Job drawing, mm, ordinate dimensions from the low corner. One solid piece. Round coordinates to 2 decimals unless told otherwise and drop trailing zeros. Write each loop counter-clockwise with the first axis right and the second up, starting at its lowest first coordinate (ties: lowest second). Pieces come first, ordered by that corner, then holes.
1) Saw through at B-B (x = 50). Write the cut outline in (y, z), plus the area to 3 significant figures.
2) Saw through at C-C (y = 89). Write the cut outline in (x, z), plus the area to 3 significant figures.
3) Wall check: probe 1 along Z at (x, y) = (19, 71.5); probe 2 along Y at (x, z) = (61.5, 37); probe 3 along Y at (x, z) = (26, 64) (1 decimal). Give the ranges that are in metal, low to high.
4) Flat gauge pins, fed straight in: pin 1 (1.8 mm diameter, centred on x = 19, y = 136.5, fed in from +Z); pin 2 (3 mm diameter, centred on x = 52.5, z = 20, fed in from -Y); pin 3 (8 mm diameter, centred on x = 26, y = 30, fed in from +Z). Where does each tip first touch, or does it go through?
5) Saw through at A-A (z = 33). Write the cut outline in (x, y), plus the area to 3 significant figures.
6) Saw through at D-D (z = 21.5). Write the cut outline in (x, y).
7) Pull direction Y, two halves, no side cores. Call the marked faces 1, 2, 3 and 4: +Y half, -Y half, draft (parallel to the pull), parting line (faces both ways), or undercut.
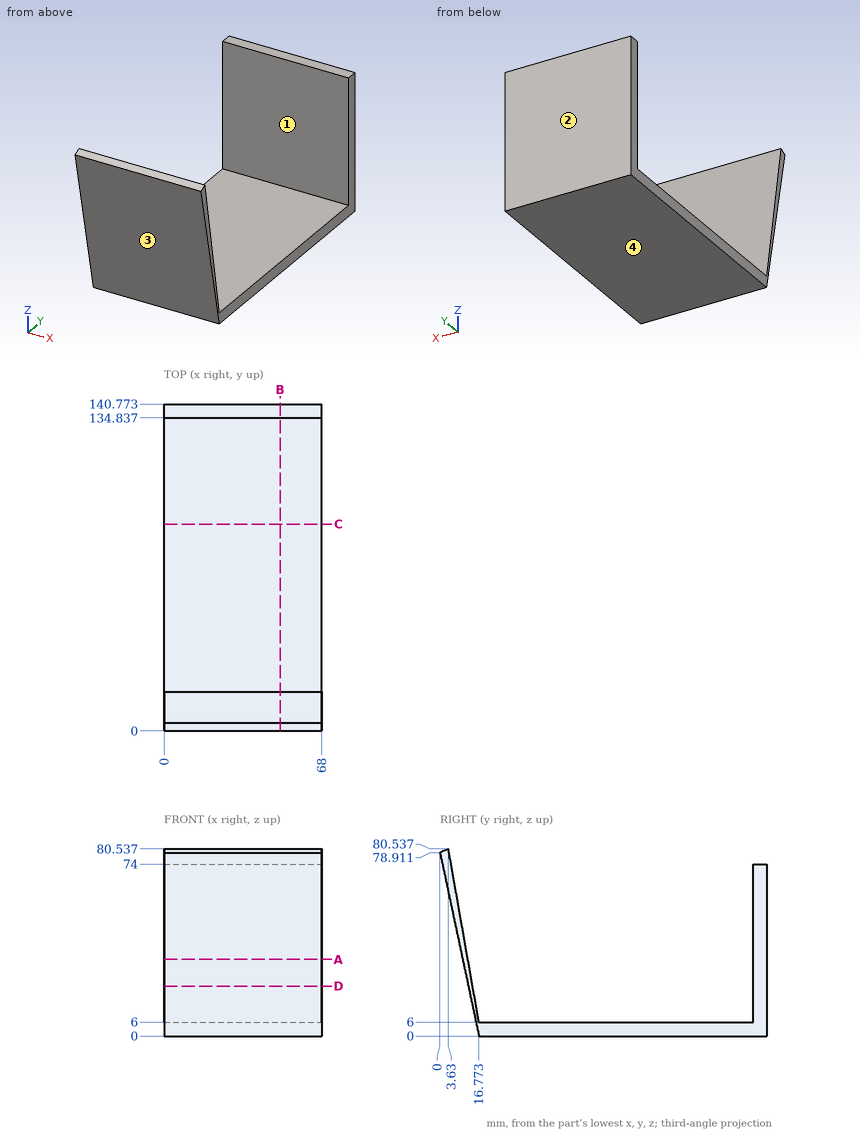
Evaluation:
1. outline: (0, 78.91) - (16.77, 0) - (140.77, 0) - (140.77, 74) - (134.84, 74) - (134.84, 6) - (16.77, 6) - (3.63, 80.54) - close
1. area: 1,340 mm2
2. outline: (0, 0) - (68, 0) - (68, 6) - (0, 6) - close
2. area: 408 mm2
3. probe 1: z = 0 to 6
3. probe 2: y = 8.91 to 11.31, 134.84 to 140.77
3. probe 3: y = 3.2 to 6.5, 134.8 to 140.8
4. pin 1: stops at z = 74
4. pin 2: stops at y = 12.2
4. pin 3: stops at z = 6
5. outline: (0, 9.76) - (68, 9.76) - (68, 12.01) - (0, 12.01) - close; (0, 134.84) - (68, 134.84) - (68, 140.77) - (0, 140.77) - close
5. area: 557 mm2
6. outline: (0, 12.2) - (68, 12.2) - (68, 14.04) - (0, 14.04) - close; (0, 134.84) - (68, 134.84) - (68, 140.77) - (0, 140.77) - close
7. face 1: undercut
7. face 2: +Y half
7. face 3: -Y half
7. face 4: draft
